Input: part model. Units: mm. Frame: model coordinates. Face numbers are marked on the shaded views. Coordinates: 2 decimals unless noted, no trailing zeros. Order: outer loops, then holes, each group sorted by start corner. A loop starts at its lowest first (then second) coordinate and runs counter-clockwise, first axis right, second up. Notation, with made-up numbers: (-14.5, 84) -> (10.5, 84) arc R6 ccw to (10.5, 93) -> close; hole circle Ø9 at (39.25, 26). An arc over 180 degrees is marked (long way). Use one line per item in the form item = value. Start each with the question number.
1) Section query C-C on z = 183. Output: boundary loops of the cut face in (x, y), then the cut area to 3 significant figures.
2) Ray query, line 1 along Y through (x, z) = (10, 23.5); line 2 along X through (y, z) = (-5.25, 177.5); line 3 along Y through (x, z) = (35.5, 131.5). Return the intervals inside material, ascending.
3) Pin query (flat end, axial travel): pin 1 (3 mm diameter, centred on y = -2, z = 83, fed in from +X); pin 2 (4 mm diameter, centred on y = -5.5, z = 179, fed in from +X); pin 3 (5 mm diameter, centred on y = -3, z = 137.5, fed in from -X). Return the tip coordinate at first contact, or that it passes through.
4) Section query D-D on x = 53. Output: boundary loops of the cut face in (y, z).
5) Draft query along X for the marked faces 1, 2 and 3. Return one class per face: pulls with the +X half, pulls with the -X half, needs draft (parallel to the pull), parting line crosses it, or undercut.
6) Section query A-A on z = 90.5. Output: boundary loops of the cut face in (x, y).
7) Section query B-B on x = 115. Output: boundary loops of the cut face in (y, z).
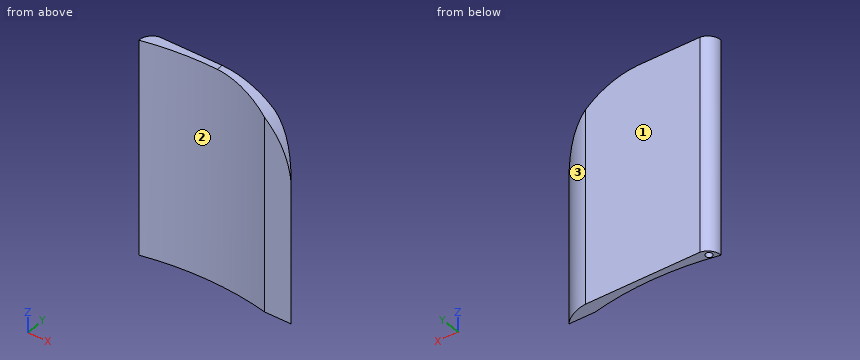
from build123d import *

# Parameters (mm, degrees)
F1_DEPTH = 12.7
F3_DEPTH = 2819.4
F4_R     = 3.175
F5_DEPTH = 44.45


with BuildPart() as f1:
    # F0 (on Front) → F1 (new body)
    with BuildSketch(Plane.XZ):
        Polygon((0, 127), (0, 0), (146.05, 0), (146.05, 131.5695), (70.539849, 208.714945), align=None)
        Polygon((0, 208.714945), (0, 127), (70.539849, 208.714945), align=None)
        with BuildLine():
            Line((70.539849, 208.714945), (146.05, 131.5695))
            ThreePointArc((146.05, 131.5695), (124.030763, 185.5445), (70.539849, 208.714945))
        make_face()
    extrude(amount=F1_DEPTH)

    # F2 (on Top) → F3 (intersect)
    with BuildSketch(Plane.XY):
        with BuildLine():
            ThreePointArc((10.757195, 0), (3.050719, -4.378233), (0, -12.7))
            ThreePointArc((0, -12.7), (60.312475, -5.995254), (120.65, -12.470686))
            Line((120.65, -12.470686), (146.05, -12.422409))
            ThreePointArc((146.05, -12.422409), (134.545033, -3.767731), (120.65, 0))
            Line((120.65, 0), (14.993685, 0))
            Line((14.993685, 0), (10.757195, 0))
        make_face()
    extrude(amount=F3_DEPTH, mode=Mode.INTERSECT)

    # F4 (on face) → F5 (cut)
    with BuildSketch(Plane(origin=(0, 0, 0), x_dir=(1, 0, 0), z_dir=(0, 0, -1))):
        with Locations((7.591504, 6.968603)):
            Circle(F4_R)
    extrude(amount=-F5_DEPTH, mode=Mode.SUBTRACT)


solid = f1.part
Answers below:
q1.outline = (0, -12.7) arc R279.4 cw to (120.65, -12.47) -> (126.41, -12.46) -> (126.41, -0.88) arc R38.1 ccw to (120.65, 0) -> (10.76, 0) arc R12.88 ccw to start
q1.area = 1,020 mm^2
q2.line_1 = -10.66 to -9.04, -4.9 to -0.15
q2.line_2 = 2.37 to 130.89
q2.line_3 = -7.15 to 0
q3.pin_1 = 133.99
q3.pin_2 = 131.26
q3.pin_3 = 2.2
q4.outline = (-6.1, 0) -> (0, 0) -> (0, 208.71) -> (-6.1, 208.71) -> close
q5.face_1 = needs draft
q5.face_2 = undercut
q5.face_3 = pulls with the +X half
q6.outline = (0, -12.7) arc R279.4 cw to (120.65, -12.47) -> (146.05, -12.42) arc R38.1 ccw to (120.65, 0) -> (10.76, 0) arc R12.88 ccw to start
q7.outline = (-11.29, 0) -> (0, 0) -> (0, 193.44) -> (-11.29, 193.44) -> close
